Geometry check sheet. Reference: the model listing, model coordinates, mm. A direction names the side the tool comes from. Give positions to 0.01 mm unless a question says otherwise; leave off trailing zeros. Loops run counter-clockwise (first coordinate to the right, second up) from the corner with the lowest first, then second, coordinate; pieces in that order, holes last. Notation, with made-up numbers: (5.25, 19) -> (37.25, 19) arc R17 cw to (37.25, 44) -> close; hole circle Ø4 at (23.25, 72.5). An arc over 180 degrees is marked (long way). One line per item, written item: value. Start each with the question number.
(1) Gauge pin test, flat ends, axial feed: pin 1 Ø1.5 at (y, z) = (-2, 11.5) entering from +X; pin 2 Ø1.2 at (x, z) = (-11.5, 1) entering from -Y; pin 3 Ø1.2 at (y, z) = (-1.5, 1) entering from -X. Record the tip position at first contact, or that the pin passes through.
(2) Draft check along X on faces 3 (the face through (0, -4, 0)), 4 (the face through (-3.848, -17.328, 0.74)), 5 (the face through (-11, -3, 1)). Enter one of: pulls with the +X half, pulls with the -X half, needs draft (parallel to the pull), parting line crosses it, or undercut.
(3) Sectioned sample at A-A, the plane y = 0. Record the cut outline in (x, z).
(4) Scan lines: line 1 along Y through (x, z) = (0, 10); line 2 along Z through (x, y) = (4, 4); line 3 along X through (y, z) = (0.5, 16). Record each from-to range of solid material in increasing order. Write a range as from..to.
(5) Sectioned sample at C-C, the plane z = 14.75. Record the cut outline in (x, y), then the cut area to 3 significant figures.
(6) Sectioned sample at B-B, the plane x = 0. Record the cut outline in (y, z).
(7) Tool access check on faces 1 (the face through (11, -3, 1)), 2 (the face through (-0.867, -3.905, 9.881)). Record the directions out of +Z, -Z, +X, -X, +Y, -Y that give a thin tool (end or side, any length) a straight path to the whole face; none if there is none.
(8) Sectioned sample at D-D, the plane y = 11. Record the cut outline in (x, z), then the cut area to 3 significant figures.
from build123d import *

# Parameters (mm, degrees)
SKETCH1_R           = 17.75
BOSS_EXTRUDE1_DEPTH = 1.5
SKETCH2_R           = 4
BOSS_EXTRUDE2_DEPTH = 17
SKETCH4_R           = 3.5
SKETCH4_W           = 3.5
SKETCH4_H           = 6
CUT_EXTRUDE1_DEPTH  = 32.182928022


with BuildPart() as part:
    # Sketch1 → Boss-Extrude1 (new body)
    with BuildSketch(Plane.XY):
        Circle(SKETCH1_R)
    extrude(amount=BOSS_EXTRUDE1_DEPTH)

    # Sketch2 → Boss-Extrude2 (add)
    with BuildSketch(Plane.XY.offset(1.5)):
        Circle(SKETCH2_R)
    extrude(amount=BOSS_EXTRUDE2_DEPTH)

    # Sketch4 → Cut-Extrude1 (cut, through all)
    with BuildSketch(Plane.XY.offset(18.5)):
        Circle(SKETCH4_R)
        with Locations((-11, 0)):
            Rectangle(SKETCH4_W, SKETCH4_H)
        with Locations((11, 0)):
            Rectangle(SKETCH4_W, SKETCH4_H)
    extrude(amount=-CUT_EXTRUDE1_DEPTH, mode=Mode.SUBTRACT)


solid = part.part
Calculated:
1. pin 1: stops at x = 3.8
1. pin 2: stops at y = -14.01
1. pin 3: stops at x = -17.73
2. face 3: needs draft
2. face 4: parting line crosses it
2. face 5: undercut
3. outline: (-17.75, 0) -> (-12.75, 0) -> (-12.75, 1.5) -> (-17.75, 1.5) -> close; (-9.25, 0) -> (-3.5, 0) -> (-3.5, 18.5) -> (-4, 18.5) -> (-4, 1.5) -> (-9.25, 1.5) -> close; (3.5, 0) -> (9.25, 0) -> (9.25, 1.5) -> (4, 1.5) -> (4, 18.5) -> (3.5, 18.5) -> close; (12.75, 0) -> (17.75, 0) -> (17.75, 1.5) -> (12.75, 1.5) -> close
4. line 1: y = -4..-3.5, 3.5..4
4. line 2: z = 0..1.5
4. line 3: x = -3.97..-3.46, 3.46..3.97
5. outline: circle Ø8 at (0, 0); hole circle Ø7 at (0, 0)
5. area: 11.8 mm2
6. outline: (-17.75, 0) -> (-3.5, 0) -> (-3.5, 18.5) -> (-4, 18.5) -> (-4, 1.5) -> (-17.75, 1.5) -> close; (3.5, 0) -> (17.75, 0) -> (17.75, 1.5) -> (4, 1.5) -> (4, 18.5) -> (3.5, 18.5) -> close
7. face 1: +Z, -Z
7. face 2: +Z
8. outline: (-13.93, 0) -> (13.93, 0) -> (13.93, 1.5) -> (-13.93, 1.5) -> close
8. area: 41.8 mm2
